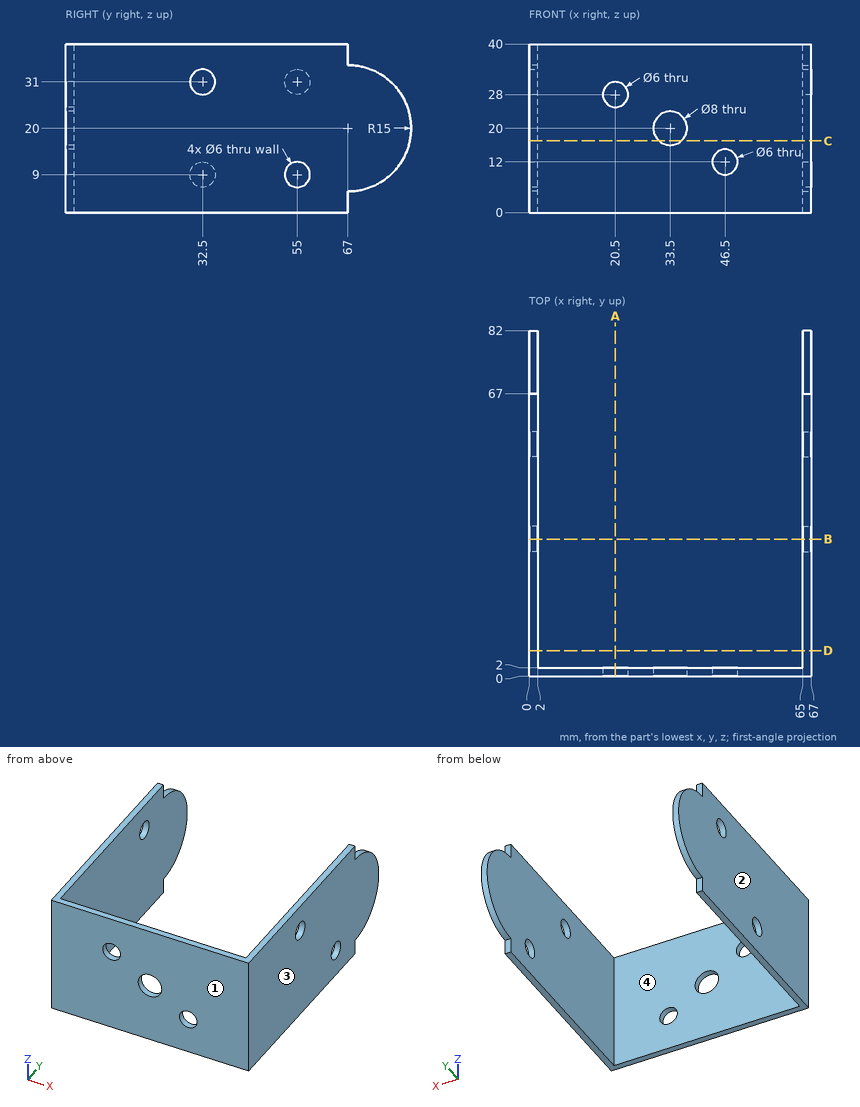
Verification items for this drawing (mm, ordinates from the low corner). Round coordinates to 2 decimals unless told otherwise and drop trailing zeros. Write each loop counter-clockwise with the first axis right and the second up, starting at its lowest first coordinate (ties: lowest second). Pieces come first, ordered by that corner, then holes. Notation, with made-up numbers: M 78,73 L 122,73 A15 cw 122,81 Z; hole C -21.75,36.5 d1. An arc over 180 degrees is marked long. Write item = value, one per line. Start each with the question number.
1. Release check for a two-part mould opening along X. For the marked faces 1, 2, 3 and 4 record: pulls with the +X half, pulls with the -X half, needs draft (parallel to the pull), parting line crosses it, or undercut.
2. Section check A-A, the plane x = 20.5. Record the cut outline in (y, z).
3. Section check D-D, the plane y = 6. Record the cut outline in (x, z), then the cut area to 3 significant figures.
4. Scan lines: line 1 (X direction, y = 61.5, z = 28); line 2 (Z direction, x = 46.5, y = 1.2); line 3 (Z direction, x = 33.5, y = 1.2). Record each from-to range of solid material in increasing order. Write a range as [from, to].
5. Gauge pin test, flat ends, axial feed: pin 1 (5 mm diameter, centred on x = 55.5, z = 35.5, fed in from +Y); pin 2 (2 mm diameter, centred on x = 65.5, z = 3.5, fed in from +Y); pin 3 (3.5 mm diameter, centred on y = 32.5, z = 9, fed in from -X); pin 4 (5 mm diameter, centred on x = 20.5, z = 28, fed in from -Y). Record the tip position at first contact, or that the pin passes through.
6. Section check C-C, the plane z = 17. Record the cut outline in (x, y), then the cut area to 3 significant figures.
7. Section check B-B, the plane y = 32.5. Record the cut outline in (x, z), then the cut area to 3 significant figures.
Results found:
q1.face_1 = needs draft
q1.face_2 = pulls with the -X half
q1.face_3 = pulls with the +X half
q1.face_4 = undercut
q2.outline = M 0,0 L 2,0 L 2,25 L 0,25 Z; M 0,31 L 2,31 L 2,40 L 0,40 Z
q3.outline = M 0,0 L 2,0 L 2,40 L 0,40 Z; M 65,0 L 67,0 L 67,40 L 65,40 Z
q3.area = 160 mm^2
q4.line_1 = [0, 2], [65, 67]
q4.line_2 = [0, 9], [15, 40]
q4.line_3 = [0, 16], [24, 40]
q5.pin_1 = 2
q5.pin_2 = 67
q5.pin_3 = 65
q5.pin_4 = through
q6.outline = M 0,0 L 30.85,0 L 30.85,2 L 2,2 L 2,81.7 L 0,81.7 Z; M 36.15,0 L 67,0 L 67,81.7 L 65,81.7 L 65,2 L 36.15,2 Z
q6.area = 442 mm^2
q7.outline = M 0,0 L 2,0 L 2,6 L 0,6 Z; M 0,12 L 2,12 L 2,40 L 0,40 Z; M 65,0 L 67,0 L 67,28 L 65,28 Z; M 65,34 L 67,34 L 67,40 L 65,40 Z
q7.area = 136 mm^2
